For this review, take the finished solid that the model builds, in its own axes (mm). Give positions to 0.01 mm unless a question says otherwise; leave off trailing zeros. Loops run counter-clockwise (first coordinate to the right, second up) from the corner with the lowest first, then second, coordinate; pieces in that order, holes last. Notation, with made-up numbers: (18.5, 65) - (59.5, 65) arc R29 ccw to (59.5, 95) - close; hole circle Ø2 at (57, 69.25). An arc over 180 degrees is marked (long way). Put each result on its own line as item: value.
from build123d import *

# Parameters (mm, degrees)
F3_R     = 5.08
F7_W     = 7.62
F7_H     = 0.7951933011
F8_DEPTH = 217.885375


with BuildPart() as f1:
    # F0 (on Top) → F1 (revolve)
    with BuildSketch(Plane.XY):
        Polygon((-19.446875, 0), (-194.865625, 0), (-194.865625, -12.7), (-169.465625, -12.7), (-169.465625, -11.1125), (-144.065625, -11.1125), (-144.065625, -9.525), (-118.665625, -9.525), (-118.665625, -5.08), (118.665625, -5.08), (118.665625, -7.9375), (144.065625, -7.9375), (144.065625, -9.525), (169.465625, -9.525), (169.465625, -6.35), (194.865625, -6.35), (194.865625, 0), align=None)
    revolve(axis=Axis((7.8748166561, 0, 0), (1, 0, 0)))

    # F4: sweep along a path in F0
    with BuildLine(Plane.XY) as f4_path:
        Line((217.884375, 73.81875), (84.2164109554, 73.81875))
        ThreePointArc((84.2164109554, 73.81875), (82.2541135698, 73.5079460533), (80.4839074509, 72.6059591245))
        Line((80.4839074509, 72.6059591245), (-19.446875, 0))
    # F3 (on plane+point) → F4 (sweep)
    with BuildSketch(Plane.YZ.offset(217.884375)):
        with Locations((73.81875, 0)):
            Circle(F3_R)
    sweep(path=f4_path.line)

    # F5 (on Top) → F6 (revolve)
    with BuildSketch(Plane.XY):
        Polygon((141.684375, 73.81875), (217.884375, 73.81875), (217.884375, 80.16875), (192.484375, 80.16875), (192.484375, 83.34375), (167.084375, 83.34375), (167.084375, 81.75625), (141.684375, 81.75625), align=None)
    revolve(axis=Axis((213.4950719774, 73.81875, 0), (1, 0, 0)))

    # F7 (on Right) → F8 (cut, through all)
    with BuildSketch(Plane.YZ):
        with Locations((0, 9.1274033494)):
            Rectangle(F7_W, F7_H)
        with Locations((0, -9.1274033494)):
            Rectangle(F7_W, F7_H)
    extrude(amount=F8_DEPTH, mode=Mode.SUBTRACT)


solid = f1.part
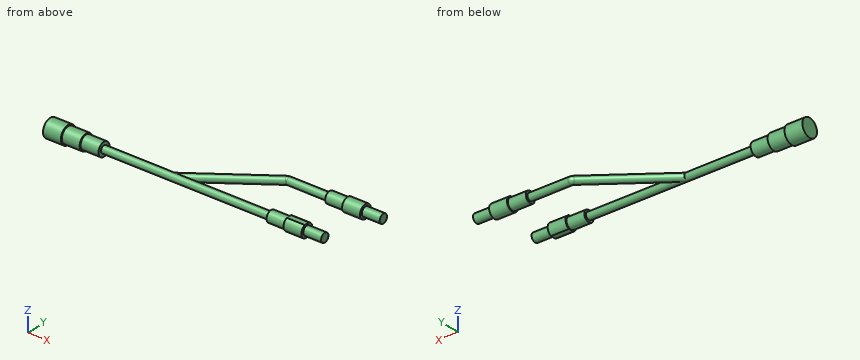
1) Insertion check: pin 1 Ø3 at (x, y) = (53.5, -1.5) entering from +Z; pin 2 Ø14 at (y, z) = (3, 2) entering from +X; pin 3 Ø4 at (y, z) = (33.5, 5.5) entering from +X; pin 4 Ø1 at (x, z) = (63.5, -6) entering from +Y. Each pin has a flat end and moves straight along its axis. Give the tip position at first contact, or say it passes through.
Geometry check:
pin 1: stops at z = 5.08
pin 2: stops at x = 194.87
pin 3: stops at x = 33.85
pin 4: passes through
2) Take a section at B-B on x = -28. State the section outline as (y, z) points.
Geometry check:
outline: circle Ø10.16 at (0, 0)
3) Take a section at A-A on x = 135.5. State the section outline as (y, z) points (1 decimal).
Geometry check:
outline: circle Ø15.9 at (0, 0); circle Ø10.2 at (73.8, 0)
4) Take a section at C-C on x = -135. State the section outline as (y, z) points (3 decimals).
Geometry check:
outline: circle Ø19.05 at (0, 0)
5) Wall thickness on line 1 (Y direction, x = 152, z = 0.25); line 2 (X direction, y = 69, z = 7.75); line 3 (X direction, y = 69.5, z = -5.5): over which ranges is each line inside the solid? List them lowest first.
Geometry check:
line 1: y = -9.52 to 9.52, 65.89 to 81.75
line 2: x = 167.08 to 192.48
line 3: x = 141.68 to 192.48
